Design review of the part built by this model. Coordinates are the model's own, in mm. Round coordinates to 2 decimals unless told otherwise and drop trailing zeros. Order: outer loops, then holes, each group sorted by start corner. A loop starts at its lowest first (then second) coordinate and runs counter-clockwise, first axis right, second up.
from build123d import *

# Parameters (mm, degrees)
BOSS_EXTRUDE1_DEPTH = 2.286
SKETCH2_R           = 2.413
CUT_EXTRUDE1_DEPTH  = 3.286
CUT_EXTRUDE2_DEPTH  = 3.286
CUT_EXTRUDE3_DEPTH  = 3.286
CIRPATTERN1_COUNT   = 3
CIRPATTERN1_ANGLE   = 90


with BuildPart() as part:
    # Sketch1 → Boss-Extrude1 (new body)
    with BuildSketch(Plane.XY):
        with BuildLine():
            Line((-42.58732985, 4.492924528), (-4.48732985, 42.545481657))
            ThreePointArc((-4.48732985, 42.545481657), (0, 44.402557128), (4.48732985, 42.545481657))
            Line((4.48732985, 42.545481657), (42.58732985, 4.492924528))
            ThreePointArc((42.58732985, 4.492924528), (43.967391701, -2.428212228), (38.1, -6.35))
            Line((38.1, -6.35), (-38.1, -6.35))
            ThreePointArc((-38.1, -6.35), (-43.967391701, -2.428212228), (-42.58732985, 4.492924528))
        make_face()
    extrude(amount=BOSS_EXTRUDE1_DEPTH)

    # Sketch2 → Cut-Extrude1 (cut, through all)
    with BuildSketch(Plane.XY.offset(2.286)):
        Circle(SKETCH2_R)
        with Locations((0, 38.052557128)):
            Circle(SKETCH2_R)
        with Locations((-25.34009434, 12.744016774)):
            Circle(SKETCH2_R)
        with Locations((25.34009434, 12.744016774)):
            Circle(SKETCH2_R)
        with Locations((-12.75990566, 25.308540354)):
            Circle(SKETCH2_R)
        with Locations((12.75990566, 25.308540354)):
            Circle(SKETCH2_R)
    extrude(amount=-CUT_EXTRUDE1_DEPTH, mode=Mode.SUBTRACT)

    # Sketch3 → Cut-Extrude2 (cut, through all)
    with BuildSketch(Plane.XY.offset(2.286)):
        with BuildLine():
            Line((-38.1, 2.413), (-12.7, 2.413))
            ThreePointArc((-12.7, 2.413), (-10.287, 0), (-12.7, -2.413))
            Line((-12.7, -2.413), (-38.1, -2.413))
            ThreePointArc((-38.1, -2.413), (-40.513, 0), (-38.1, 2.413))
        make_face()
    cut_extrude2 = extrude(amount=-CUT_EXTRUDE2_DEPTH, mode=Mode.SUBTRACT)

    # Mirror1: Cut-Extrude2 across plane
    add(cut_extrude2.mirror(Plane(origin=(0, 0, 0), x_dir=(0, 0, 1), z_dir=(1, 0, 0))), mode=Mode.SUBTRACT)

    # Sketch4 → Cut-Extrude3 (cut, through all)
    with BuildSketch(Plane.XY.offset(2.286)):
        with BuildLine():
            Line((-20.745443214, 17.33294655), (-10.69382435, 7.268795606))
            ThreePointArc((-10.69382435, 7.268795606), (-7.281327686, 7.266669629), (-7.279201708, 10.679166292))
            Line((-7.279201708, 10.679166292), (-17.330820572, 20.743317236))
            ThreePointArc((-17.330820572, 20.743317236), (-20.743317236, 20.745443214), (-20.745443214, 17.33294655))
        make_face()
    cut_extrude3 = extrude(amount=-CUT_EXTRUDE3_DEPTH, mode=Mode.SUBTRACT)

    # CirPattern1: Cut-Extrude3 ×3 about axis
    cirpattern1_axis = Axis((0, 0, 0), (0, 0, -1))
    for i in range(1, CIRPATTERN1_COUNT):
        add(cut_extrude3.rotate(cirpattern1_axis, i * CIRPATTERN1_ANGLE / (CIRPATTERN1_COUNT - 1)), mode=Mode.SUBTRACT)


solid = part.part
1) Clearance check with flat-ended pins moving along their axes: P1, Ø4.5, axis at x = 25.34, y = 12.74, coming from the -Z side; P2, Ø1.1, axis at x = -21, z = 1.5, coming from the +Y side. State where each tip first meets the part, or that it passes through.
Results:
P1: passes through
P2: stops at y = 26.6
2) Take a section at D-D on y = 14. Give the boundary of the cut face in (x, z), plus the area to 3 significant figures.
Results:
outline: (-33.07, 0) - (-27.4, 0) - (-27.4, 2.29) - (-33.07, 2.29) - close; (-23.28, 0) - (-17.42, 0) - (-17.42, 2.29) - (-23.28, 2.29) - close; (-10.6, 0) - (-2.42, 0) - (-2.42, 2.29) - (-10.6, 2.29) - close; (2.4, 0) - (10.58, 0) - (10.58, 2.29) - (2.4, 2.29) - close; (17.41, 0) - (23.28, 0) - (23.28, 2.29) - (17.41, 2.29) - close; (27.4, 0) - (33.07, 0) - (33.07, 2.29) - (27.4, 2.29) - close
area: 90.1 mm2
3) The part is to be moulded in two halves that separate along X. For faces 1 (the face through (-25, -2.413, 1)), 2 (the face through (-23.804, 23.253, 1.127)), say which applies: released by +X, released by -X, zero draft, split by the parting line, or undercut.
Results:
face 1: undercut
face 2: released by -X
4) Take a section at B-B on x = 30.5. Give the boundary of the cut face in (y, z), plus the area to 3 significant figures.
Results:
outline: (-6.35, 0) - (-2.41, 0) - (-2.41, 2.29) - (-6.35, 2.29) - close; (2.41, 0) - (16.57, 0) - (16.57, 2.29) - (2.41, 2.29) - close
area: 41.4 mm2
5) To check wall thickness, follow line 1 along Y through (x, z) = (0, 1.5); line 2 along Y through (x, z) = (-20, 1.2); line 3 along X through (y, z) = (10, 0.25). State the ranges of each line that lie inside material, in increasing order.
Results:
line 1: y = -6.35 to -2.41, 2.41 to 10.29, 29.34 to 35.64, 40.47 to 44.4
line 2: y = -6.35 to -2.41, 2.41 to 16.59, 21.25 to 27.05
line 3: x = -37.07 to -13.42, -6.8 to 6.78, 13.4 to 37.07
6) Take a section at C-C on z = 1.75. State how many separate pieces and enclosed holes the cut face has, plus the area to 3 significant figures.
Results:
separate pieces: 1
enclosed holes: 11
area: 2,090 mm2
7) Take a section at A-A on y = 0. Give the boundary of the cut face in (x, z).
Results:
outline: (-44.45, 0) - (-40.51, 0) - (-40.51, 2.29) - (-44.45, 2.29) - close; (-10.29, 0) - (-2.41, 0) - (-2.41, 2.29) - (-10.29, 2.29) - close; (2.41, 0) - (10.29, 0) - (10.29, 2.29) - (2.41, 2.29) - close; (40.51, 0) - (44.45, 0) - (44.45, 2.29) - (40.51, 2.29) - close
